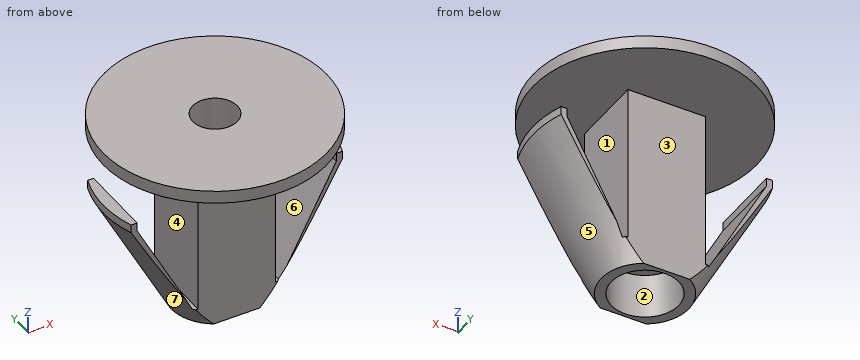
from build123d import *

# Parameters (mm, degrees)
CUT_EXTRUDE1_DEPTH      = 8.5
CUT_EXTRUDE1_DEPTH_BACK = 8.5
CUT_EXTRUDE3_DEPTH      = 8.5
CUT_EXTRUDE3_DEPTH_BACK = 8.5
CUT_EXTRUDE4_DEPTH      = 8.5
CUT_EXTRUDE4_DEPTH_BACK = 8.5
SKETCH6_R               = 1.5
CUT_EXTRUDE5_DEPTH      = 8.830238334
CUT_EXTRUDE5_DEPTH_BACK = 6.169761666
SKETCH8_R               = 2.264503928
CUT_EXTRUDE6_DEPTH      = 3


with BuildPart() as part:
    # Sketch2 → Revolve1 (revolve)
    with BuildSketch(Plane(origin=(0, 0, 0), x_dir=(1, 0, 0), z_dir=(0, 1, 0))):
        Polygon((0, 5.169761666), (-2.93214923, 5.169761666), (-7.5, -3.499678513), (-7.5, -7.830238334), (0, -7.830238334), align=None)
    revolve(axis=Axis((0, 0, 7.830238334), (0, 0, -1)))

    # Sketch3 → Cut-Extrude1 (cut, two sides)
    with BuildSketch(Plane(origin=(0, 0, 0), x_dir=(1, 0, 0), z_dir=(0, 1, 0))) as cut_extrude1_sk:
        Polygon((-7.696381126, -4.06313473), (-4.427121887, -4.06313473), (-4.427121887, -6.974818739), (-8.445586368, -6.974818739), align=None)
        Polygon((8.445586368, -6.974818739), (7.696381126, -4.06313473), (4.427121887, -4.06313473), (4.427121887, -6.974818739), align=None)
    extrude(amount=CUT_EXTRUDE1_DEPTH, mode=Mode.SUBTRACT)
    extrude(cut_extrude1_sk.sketch, amount=-CUT_EXTRUDE1_DEPTH_BACK, mode=Mode.SUBTRACT)

    # Sketch4 → Cut-Extrude3 (cut, two sides)
    with BuildSketch(Plane(origin=(0, 0, 0), x_dir=(1, 0, 0), z_dir=(0, 1, 0))) as cut_extrude3_sk:
        Polygon((-6.673039702, -4.06313473), (-6.673039702, -3.499678513), (-2.88374221, 3.692125592), (-2.603089552, 3.692125592), (-2.603089552, -4.06313473), (-2.603089552, -6.974818739), (-6.673039702, -6.974818739), align=None)
        Polygon((2.603089552, -6.974818739), (2.603089552, -4.06313473), (2.603089552, 3.692125592), (2.88374221, 3.692125592), (6.673039702, -3.499678513), (6.673039702, -4.06313473), (6.673039702, -6.974818739), align=None)
    extrude(amount=CUT_EXTRUDE3_DEPTH, mode=Mode.SUBTRACT)
    extrude(cut_extrude3_sk.sketch, amount=-CUT_EXTRUDE3_DEPTH_BACK, mode=Mode.SUBTRACT)

    # Sketch5 → Cut-Extrude4 (cut, two sides)
    with BuildSketch(Plane(origin=(0, 0, 0), x_dir=(0, 0, -1), z_dir=(1, 0, 0))) as cut_extrude4_sk:
        Polygon((-6.974818739, 2.495248244), (8.7529713, 2.495248244), (-4.227454646, 9.024441475), (-6.974818739, 9.024441475), align=None)
        Polygon((-6.974818739, -9.024441475), (-6.974818739, -2.495248244), (8.7529713, -2.495248244), (-4.227454646, -9.024441475), align=None)
    extrude(amount=CUT_EXTRUDE4_DEPTH, mode=Mode.SUBTRACT)
    extrude(cut_extrude4_sk.sketch, amount=-CUT_EXTRUDE4_DEPTH_BACK, mode=Mode.SUBTRACT)

    # Sketch6 → Cut-Extrude5 (cut, two sides)
    with BuildSketch(Plane.XY) as cut_extrude5_sk:
        Circle(SKETCH6_R)
    extrude(amount=CUT_EXTRUDE5_DEPTH, mode=Mode.SUBTRACT)
    extrude(cut_extrude5_sk.sketch, amount=-CUT_EXTRUDE5_DEPTH_BACK, mode=Mode.SUBTRACT)

    # Sketch8 → Cut-Extrude6 (cut)
    with BuildSketch(Plane(origin=(0, 0, -5.169761666), x_dir=(-1, 0, 0), z_dir=(0, 0, -1))):
        Circle(SKETCH8_R)
    extrude(amount=-CUT_EXTRUDE6_DEPTH, mode=Mode.SUBTRACT)


solid = part.part
Could you check a few things on this model? Use its own coordinates, in mm. Face numbers are marked on the shaded views. A direction names the side the tool comes from. Give positions to 0.01 mm unless a question says otherwise; leave off trailing zeros. Order: outer loops, then holes, each group sorted by start corner. A loop starts at its lowest first (then second) coordinate and runs counter-clockwise, first axis right, second up. Notation, with made-up numbers: (17.5, -6.75) - (49.5, -6.75) arc R10 ccw to (49.5, 8.25) - close; hole circle Ø11 at (23, 17). An arc over 180 degrees is marked (long way). One line per question, with ' | ' between items. Start each with the question number.
Item 1: I want a section at B-B on z = 2.75. Write out the boundary of the cut face in (x, y) (3 decimals).
Item 2: Thinking about a two-plate mould opening in X: for the marked faces 4, 5, 6 and 7, which applies, pulls with the +X half, pulls with the -X half, needs draft (parallel to the pull), parting line crosses it, or undercut?
Item 3: For the marked faces 1, 2 and 3, which set-ups out of +Z, -Z, +X, -X, +Y, -Y let a thin tool reach every point of the face, with its end or its side?
Item 4: I want a section at C-C on x = 0. Write out the boundary of the cut face in (y, z).
Item 5: I need wall thicknesses on probe 1 along Y at (x, z) = (0, 2); probe 2 along X at (y, z) = (0.25, -3.25); probe 3 along X at (y, z) = (0, 6). Which ranges of each line are inside material? Lowest first, please. Write a range as [from, to].
Item 6: I'm going to push flat-ended pins straight in: pin 1 Ø1 at (y, z) = (4.5, -1.5) entering from +X; pin 2 Ø4 at (x, z) = (-5, 2) entering from -Y; pin 3 Ø1.9 at (x, z) = (-4.5, 0.5) entering from +Y; pin 4 Ø3 at (y, z) = (3, -3.5) entering from -X. Where does each tip first touch, or does it pass through?
Item 7: I want a section at D-D on z = 6. Write out the boundary of the cut face in (x, y).
Item 8: I want a section at A-A on y = 0. Write out the boundary of the cut face in (x, z), then the cut area to 3 significant figures.
Verdict:
1) outline: (-6.652, -2.495) - (-6.278, -2.495) - (-6.278, 2.495) - (-6.652, 2.495) arc R7.105 ccw to start; (-2.603, -2.495) - (2.603, -2.495) - (2.603, 2.495) - (-2.603, 2.495) - close; (6.278, -2.495) - (6.652, -2.495) arc R7.105 ccw to (6.652, 2.495) - (6.278, 2.495) - close; hole circle Ø3 at (0, 0)
2) face 4: undercut | face 5: pulls with the +X half | face 6: undercut | face 7: pulls with the -X half
3) face 1: +Y, -Y | face 2: -Z | face 3: -Z, +X, -X, +Y
4) outline: (-7.5, 6.97) - (-2.5, 6.97) - (-2.5, -5.17) - (-2.26, -5.17) - (-2.26, -2.17) - (-1.5, -2.17) - (-1.5, 7.83) - (-7.5, 7.83) - close; (1.5, -2.17) - (2.26, -2.17) - (2.26, -5.17) - (2.5, -5.17) - (2.5, 6.97) - (7.5, 6.97) - (7.5, 7.83) - (1.5, 7.83) - close
5) probe 1: [-2.5, -1.5], [1.5, 2.5] | probe 2: [-3.94, -3.12], [-2.6, -2.25], [2.25, 2.6], [3.12, 3.94] | probe 3: [-2.6, -1.5], [1.5, 2.6]
6) pin 1: through | pin 2: y = -2.5 | pin 3: y = 2.5 | pin 4: x = -3.92
7) outline: (-2.6, -2.5) - (2.6, -2.5) - (2.6, 2.5) - (-2.6, 2.5) - close; hole circle Ø3 at (0, 0)
8) outline: (-7.5, 3.5) - (-2.93, -5.17) - (-2.26, -5.17) - (-2.26, -2.17) - (-1.5, -2.17) - (-1.5, 7.83) - (-7.5, 7.83) - (-7.5, 6.97) - (-2.6, 6.97) - (-2.6, -3.69) - (-2.88, -3.69) - (-6.67, 3.5) - (-6.67, 4.06) - (-7.5, 4.06) - close; (1.5, -2.17) - (2.26, -2.17) - (2.26, -5.17) - (2.93, -5.17) - (7.5, 3.5) - (7.5, 4.06) - (6.67, 4.06) - (6.67, 3.5) - (2.88, -3.69) - (2.6, -3.69) - (2.6, 6.97) - (7.5, 6.97) - (7.5, 7.83) - (1.5, 7.83) - close | area: 47.4 mm^2
